```python
from build123d import *

# Parameters (mm, degrees)
BOSS_EXTRUDE1_DEPTH = 20
CUT_EXTRUDE1_REACH  = 36.478
SKETCH3_R           = 1.5


with BuildPart() as part:
    # Sketch1 → Boss-Extrude1 (new body)
    with BuildSketch(Plane.XY):
        with BuildLine():
            Line((8.135150199, -2.180546666), (-4.364849801, -2.180546666))
            Line((-4.364849801, -2.180546666), (-4.364849801, 2.819453334))
            Line((-4.364849801, 2.819453334), (27.635150199, 2.819453334))
            Line((27.635150199, 2.819453334), (27.635150199, -2.180546666))
            Line((27.635150199, -2.180546666), (15.135150199, -2.180546666))
            ThreePointArc((15.135150199, -2.180546666), (11.635150199, 1.319453334), (8.135150199, -2.180546666))
        make_face()
    extrude(amount=BOSS_EXTRUDE1_DEPTH)

    # Sketch3 → Cut-Extrude1 (cut, up to next)
    with BuildSketch(Plane.XZ.offset(2.180546666), mode=Mode.PRIVATE) as cut_extrude1_sk1:
        with Locations((-1.364849801, 15)):
            Circle(SKETCH3_R)
    cut_extrude1_tool1 = extrude(cut_extrude1_sk1.sketch, amount=-CUT_EXTRUDE1_REACH, mode=Mode.PRIVATE) & part.part
    # Sketch3 → Cut-Extrude1 (cut, up to next)
    with BuildSketch(Plane.XZ.offset(2.180546666), mode=Mode.PRIVATE) as cut_extrude1_sk2:
        with Locations((-1.364849801, 5)):
            Circle(SKETCH3_R)
    cut_extrude1_tool2 = extrude(cut_extrude1_sk2.sketch, amount=-CUT_EXTRUDE1_REACH, mode=Mode.PRIVATE) & part.part
    # Sketch3 → Cut-Extrude1 (cut, up to next)
    with BuildSketch(Plane.XZ.offset(2.180546666), mode=Mode.PRIVATE) as cut_extrude1_sk3:
        with Locations((24.635150199, 15)):
            Circle(SKETCH3_R)
    cut_extrude1_tool3 = extrude(cut_extrude1_sk3.sketch, amount=-CUT_EXTRUDE1_REACH, mode=Mode.PRIVATE) & part.part
    # Sketch3 → Cut-Extrude1 (cut, up to next)
    with BuildSketch(Plane.XZ.offset(2.180546666), mode=Mode.PRIVATE) as cut_extrude1_sk4:
        with Locations((24.635150199, 5)):
            Circle(SKETCH3_R)
    cut_extrude1_tool4 = extrude(cut_extrude1_sk4.sketch, amount=-CUT_EXTRUDE1_REACH, mode=Mode.PRIVATE) & part.part
    add(cut_extrude1_tool1.solids().sort_by_distance((-1.36485, -2.180547, 15))[0], mode=Mode.SUBTRACT)
    add(cut_extrude1_tool2.solids().sort_by_distance((-1.36485, -2.180547, 5))[0], mode=Mode.SUBTRACT)
    add(cut_extrude1_tool3.solids().sort_by_distance((24.63515, -2.180547, 15))[0], mode=Mode.SUBTRACT)
    add(cut_extrude1_tool4.solids().sort_by_distance((24.63515, -2.180547, 5))[0], mode=Mode.SUBTRACT)


solid = part.part
```
Here's how the part is built. I have some questions about the finished solid (model axes, mm). Give positions to 0.01 mm unless a question says otherwise; leave off trailing zeros. Write each loop counter-clockwise with the first axis right and the second up, starting at its lowest first coordinate (ties: lowest second). Pieces come first, ordered by that corner, then holes.
(1) Will this pin go through, and if not, where does the flat tip stop? pin 1 (2.5 mm diameter, centred on x = -1.36, z = 5, fed in from +Y).
Output values:
pin 1: passes through
(2) Thinking about a two-plate mould opening in Z: for faces 1 (the face through (11.9, 1.5, 0)), 2 (the face through (11, 2.819, 10)), 3 (the face through (-2.47, 0.284, 16.014)), which applies, pulls with the +Z half, pulls with the -Z half, needs draft (parallel to the pull), parting line crosses it, or undercut?
Output values:
face 1: pulls with the -Z half
face 2: needs draft
face 3: undercut
(3) Imagine slicing it at A-A, the plane z = 15. Write out the boundary of the cut face in (x, y), and give its area (3 significant figures).
Output values:
outline: (-4.36, -2.18) - (-2.86, -2.18) - (-2.86, 2.82) - (-4.36, 2.82) - close; (0.14, -2.18) - (8.14, -2.18) arc R3.5 cw to (15.14, -2.18) - (23.14, -2.18) - (23.14, 2.82) - (0.14, 2.82) - close; (26.14, -2.18) - (27.64, -2.18) - (27.64, 2.82) - (26.14, 2.82) - close
area: 111 mm2
(4) If I drill on L1, parallel to Z at x = 24, y = 1.5; L2, parallel to Z at x = 26, y = -0.95; L3, parallel to X at y = -1.7, z = 3.25, over which ranges is the centre line in solid material (lowest first)?
Output values:
L1: z = 0 to 3.64, 6.36 to 13.64, 16.36 to 20
L2: z = 0 to 4.38, 5.62 to 14.38, 15.62 to 20
L3: x = -4.36 to 8.17, 15.1 to 27.64
(5) Imagine slicing it at C-C, the plane z = 2.25. Write out the boundary of the cut face in (x, y).
Output values:
outline: (-4.36, -2.18) - (8.14, -2.18) arc R3.5 cw to (15.14, -2.18) - (27.64, -2.18) - (27.64, 2.82) - (-4.36, 2.82) - close
(6) Imagine slicing it at D-D, the plane y = 0.75. Write out the boundary of the cut face in (x, z), and give its area (3 significant figures).
Output values:
outline: (-4.36, 0) - (9.72, 0) - (9.72, 20) - (-4.36, 20) - close; (13.55, 0) - (27.64, 0) - (27.64, 20) - (13.55, 20) - close; hole circle Ø3 at (-1.36, 5); hole circle Ø3 at (-1.36, 15); hole circle Ø3 at (24.64, 5); hole circle Ø3 at (24.64, 15)
area: 535 mm2
(7) Imagine slicing it at B-B, the plane y = -0.75. Write out the boundary of the cut face in (x, z).
Output values:
outline: (-4.36, 0) - (8.44, 0) - (8.44, 20) - (-4.36, 20) - close; (14.83, 0) - (27.64, 0) - (27.64, 20) - (14.83, 20) - close; hole circle Ø3 at (-1.36, 5); hole circle Ø3 at (-1.36, 15); hole circle Ø3 at (24.64, 5); hole circle Ø3 at (24.64, 15)
